Geometry check sheet. Reference: the model listing, model coordinates, mm. Round coordinates to 2 decimals unless told otherwise and drop trailing zeros. Loops run counter-clockwise (first coordinate to the right, second up) from the corner with the lowest first, then second, coordinate; pieces in that order, holes last.
```python
from build123d import *

# Parameters (mm, degrees)
SKETCH1_W           = 2
SKETCH1_H           = 0.732050808
SKETCH1_W_2         = 0.732050808
SKETCH1_H_2         = 2
BOSS_EXTRUDE1_DEPTH = 22
SKETCH2_R           = 2
BOSS_EXTRUDE2_DEPTH = 9
SKETCH3_R           = 2.5
BOSS_EXTRUDE3_DEPTH = 0.5
FILLET1_R           = 0.5
FILLET2_R           = 0.1


with BuildPart() as part:
    # Sketch1 → Boss-Extrude1 (new body)
    with BuildSketch(Plane(origin=(0, 0, 0), x_dir=(1, 0, 0), z_dir=(0, 1, 0))):
        with BuildLine():
            Line((-1, 1.732050808), (1, 1.732050808))
            ThreePointArc((1, 1.732050808), (0, 2), (-1, 1.732050808))
        make_face()
        with Locations((0, 1.366025404)):
            Rectangle(SKETCH1_W, SKETCH1_H)
        with BuildLine():
            Line((1.732050808, -1), (1.732050808, 1))
            ThreePointArc((1.732050808, 1), (2, 0), (1.732050808, -1))
        make_face()
        with Locations((1.366025404, 0)):
            Rectangle(SKETCH1_W_2, SKETCH1_H_2)
        Rectangle(SKETCH1_W, SKETCH1_H_2)
        with Locations((-1.366025404, 0)):
            Rectangle(SKETCH1_W_2, SKETCH1_H_2)
        with BuildLine():
            Line((-1.732050808, -1), (-1.732050808, 1))
            ThreePointArc((-1.732050808, 1), (-2, 0), (-1.732050808, -1))
        make_face()
        with Locations((0, -1.366025404)):
            Rectangle(SKETCH1_W, SKETCH1_H)
        with BuildLine():
            Line((-1, -1.732050808), (1, -1.732050808))
            ThreePointArc((1, -1.732050808), (0, -2), (-1, -1.732050808))
        make_face()
    extrude(amount=BOSS_EXTRUDE1_DEPTH)

    # Sketch2 → Boss-Extrude2 (add)
    with BuildSketch(Plane.XZ):
        with Locations(Location((0, 0, 0), (0, 0, 270))):
            Circle(SKETCH2_R)
    extrude(amount=BOSS_EXTRUDE2_DEPTH)

    # Sketch3 → Boss-Extrude3 (add)
    with BuildSketch(Plane.XZ.offset(9)):
        with Locations(Location((0, 0, 0), (0, 0, 270))):
            Circle(SKETCH3_R)
    extrude(amount=-BOSS_EXTRUDE3_DEPTH)

    # Fillet1
    fillet1_edges = [part.edges().sort_by_distance(p)[0] for p in [
        (-1, 22, -1.366025404),
        (-1.366025404, 22, -1),
        (-2, 22, 0),
        (-1.366025404, 22, 1),
        (-1, 22, 1.366025404),
        (0, 22, 2),
        (1, 22, 1.366025404),
        (1.366025404, 22, 1),
        (0, 22, -2),
        (2, 22, 0),
        (1.366025404, 22, -1),
        (1, 22, -1.366025404),
    ]]
    fillet(fillet1_edges, radius=FILLET1_R)

    # Fillet2
    fillet2_edges = [part.edges().sort_by_distance(p)[0] for p in [
        (0, -8.5, 2),
    ]]
    fillet(fillet2_edges, radius=FILLET2_R)


solid = part.part
```
1) Sectioned sample at B-B, the plane z = 0. Record the cut outline in (x, y), then the cut area to 3 significant figures.
Report:
outline: (-2.5, -9) - (2.5, -9) - (2.5, -8.5) - (2.1, -8.5) arc R0.1 cw to (2, -8.4) - (2, 21.5) arc R0.5 ccw to (1.5, 22) - (-1.5, 22) arc R0.5 ccw to (-2, 21.5) - (-2, -8.4) arc R0.1 cw to (-2.1, -8.5) - (-2.5, -8.5) - close
area: 124 mm2
2) Gauge pin test, flat ends, axial feed: pin 1 (0.6 mm diameter, centred on y = 14, z = -1.5, fed in from -X); pin 2 (0.8 mm diameter, centred on x = -1.5, z = 1.5, fed in from +Y); pin 3 (0.8 mm diameter, centred on x = -1.5, y = 8, fed in from +Z). Record the tip position at first contact, or that the pin passes through.
Report:
pin 1: stops at x = -1
pin 2: stops at y = 0
pin 3: stops at z = 1
3) Scan lines: line 1 along Z through (x, y) = (0.1, -1.5); line 2 along Y through (x, z) = (2.25, -0.25); line 3 along Z through (x, y) = (1.5, 16). Record each from-to range of solid material in increasing order.
Report:
line 1: z = -2 to 2
line 2: y = -9 to -8.5
line 3: z = -1 to 1
4) Sectioned sample at A-A, the plane y = 9. Record the cut outline in (x, z), then the cut area to 3 significant figures.
Report:
outline: (-1.73, -1) - (-1, -1) - (-1, -1.73) arc R2 ccw to (1, -1.73) - (1, -1) - (1.73, -1) arc R2 ccw to (1.73, 1) - (1, 1) - (1, 1.73) arc R2 ccw to (-1, 1.73) - (-1, 1) - (-1.73, 1) arc R2 ccw to start
area: 11.3 mm2
